from build123d import *

# Parameters (mm, degrees)
SKETCH1_R               = 40.5
BOSS_EXTRUDE1_DEPTH     = 6
SKETCH2_W               = 40
SKETCH2_H               = 48
FILLET1_R               = 12
SKETCH4_R               = 16
BOSS_EXTRUDE2_DEPTH     = 34
SKETCH5_R               = 3.5
CUT_EXTRUDE1_DEPTH      = 15.0000001
CUT_EXTRUDE1_DEPTH_BACK = 41


with BuildPart() as part:
    # Sketch1 → Boss-Extrude1 (new body)
    with BuildSketch(Plane.XY):
        Circle(SKETCH1_R)
    extrude(amount=BOSS_EXTRUDE1_DEPTH)

    # Sweep1: sweep along a path in Sketch3
    with BuildLine(Plane.XY.offset(-24)) as sweep1_path:
        CenterArc((0, 0), 70, 0, 360)
    # Sketch2 → Sweep1 (sweep)
    with BuildSketch(Plane(origin=(0, 0, 0), x_dir=(1, 0, 0), z_dir=(0, 1, 0))):
        with Locations((36, 24)):
            Rectangle(SKETCH2_W, SKETCH2_H)
    sweep(path=sweep1_path.line)

    # Fillet1
    fillet1_edges = [part.edges().sort_by_distance(p)[0] for p in [
        (-16, 0, -48),
        (-56, 0, -48),
        (-56, 0, 0),
    ]]
    fillet(fillet1_edges, radius=FILLET1_R)

    # Sketch4 → Boss-Extrude2 (add)
    with BuildSketch(Plane(origin=(0, 0, 0), x_dir=(-1, 0, 0), z_dir=(0, 0, -1))):
        Circle(SKETCH4_R)
    extrude(amount=BOSS_EXTRUDE2_DEPTH)

    # Sketch5 → Cut-Extrude1 (cut, two sides)
    with BuildSketch(Plane(origin=(0, 0, -34), x_dir=(-1, 0, 0), z_dir=(0, 0, -1))) as cut_extrude1_sk:
        Circle(SKETCH5_R)
    extrude(amount=CUT_EXTRUDE1_DEPTH, mode=Mode.SUBTRACT)
    extrude(cut_extrude1_sk.sketch, amount=-CUT_EXTRUDE1_DEPTH_BACK, mode=Mode.SUBTRACT)


solid = part.part
Design review of the part built by this model. Coordinates are the model's own, in mm. A direction names the side the tool comes from. Round coordinates to 2 decimals unless told otherwise and drop trailing zeros. Write each loop counter-clockwise with the first axis right and the second up, starting at its lowest first coordinate (ties: lowest second). Pieces come first, ordered by that corner, then holes. Notation, with made-up numbers: (55.5, 81.5) - (110.5, 81.5) arc R18 cw to (110.5, 109.5) - close; hole circle Ø8 at (4, 48). An arc over 180 degrees is marked (long way). Use a Markdown table: item, result. Add a question column.
1. Clearance check with flat-ended pins moving along their axes: pin 1 (8 mm diameter, centred on x = -26, z = -15.5, fed in from +Y); pin 2 (2 mm diameter, centred on y = 12, z = -38.5, fed in from +X); pin 3 (9.5 mm diameter, centred on x = -2, y = 5.5, fed in from -Z). State where each tip first meets the part, or that it passes through.
2. For faces 5 (the face through (0, 4, -34)), 6 (the face through (51.73, -21.45, -24.17)), list the 3-axis set-ups (+Z, -Z, +X, -X, +Y, -Y) from which the entire face can be reached by the end or side of a thin tool; tool diameter is ignored.
3. We need section A-A (z = -32). State the section outline as (x, y) points.
4. Wall thickness on probe 1 along Y at (x, z) = (0, -34.9); probe 2 along Y at (x, z) = (0, -25.5); probe 3 along Z at (x, y) = (-40.5, -18): over which ranges is each line inside the solid? List them lowest first.
5. Mouldability with a two-part tool opening along X and no side actions: class faces 1 (the face through (21.77, 34.15, 2.96)), 2 (the face through (-3.233, -1.341, -14.28)), 3 (the face through (14.78, -6.13, -34.99)), 4 (the face through (-1, -8, 6)) as +X half, -X half, draft (parallel to the pull), parting line (faces both ways), or undercut.
Output:
| question | item | result |
|---|---|---|
| 1 | pin 1 | stops at y = 51.5 |
| 1 | pin 2 | stops at x = 54.71 |
| 1 | pin 3 | stops at z = -34 |
| 2 | face 5 | -Z |
| 2 | face 6 | +Z, -Z |
| 3 | outline | circle Ø112 at (0, 0); hole circle Ø7 at (0, 0) |
| 4 | probe 1 | y = -56 to -16, 16 to 56 |
| 4 | probe 2 | y = -56 to -3.5, 3.5 to 56 |
| 4 | probe 3 | z = -48 to 0 |
| 5 | face 1 | parting line |
| 5 | face 2 | undercut |
| 5 | face 3 | undercut |
| 5 | face 4 | draft |
